The listing builds one solid part. Answer for the finished solid, in the listing's coordinates (mm). Face numbers are marked on the shaded views. Coordinates: 2 decimals unless noted, no trailing zeros. Order: outer loops, then holes, each group sorted by start corner. A loop starts at its lowest first (then second) coordinate and runs counter-clockwise, first axis right, second up. Notation, with made-up numbers: (38, 20.5) - (61, 20.5) arc R31 ccw to (61, 47.5) - close; hole circle Ø9 at (56, 36.5). An arc over 180 degrees is marked (long way). Use a Markdown table: item, result. Add a question column.
Item 1: The part is cut by section C-C, the plane y = -1.5. Give the vertices of the cut face in (x, z).
Item 2: The part is cut by section B-B, the plane x = 2.5. Give the vertices of the cut face in (y, z), then the cut area to 3 significant figures.
Item 3: Find the intervals of material crossed by line 1 along X through (y, z) = (-3.25, 9.5); line 2 along X through (y, z) = (-1, -2); line 3 along Y through (x, z) = (-2.75, 10.25), in increasing order.
Item 4: The part is cut by section D-D, the plane z = -1.5. Give the vertices of the cut face in (x, y), then the cut area to 3 significant figures.
Item 5: The mould has two halves that part along Z. Classify the marked faces 1, 2 and 3: released by +Z, released by -Z, zero draft, split by the parting line, or undercut.
Item 6: Flat-ended cylindrical pins translate along their axes: P1, Ø2, axis at y = -2, z = 0, coming from the +X side; P2, Ø1.6, axis at x = 5, y = -0.5, coming from the +Z side; P3, Ø4, axis at y = -2.5, z = 5, coming from the -X side. Find the tip coordinate at first contact, or state that the pin passes through.
Item 7: The part is cut by section A-A, the plane z = 11.75. Give the vertices of the cut face in (x, y).
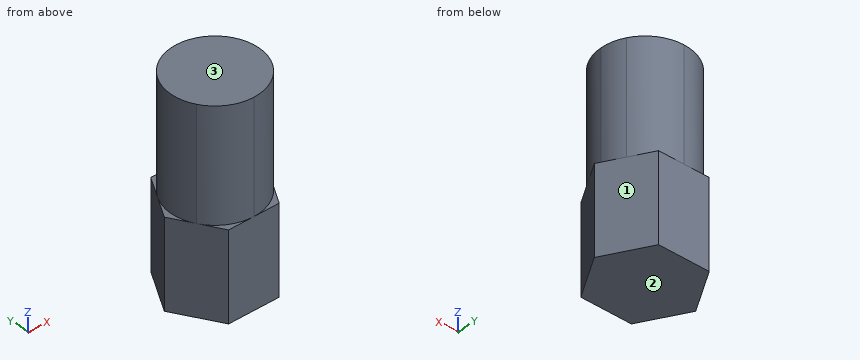
from build123d import *

# Parameters (mm, degrees)
F1_DEPTH = 5.0038
F3_DEPTH = 12.7


with BuildPart() as f1:
    # F0 (on Top) → F1 (new body, symmetric)
    with BuildSketch(Plane.XY):
        Polygon((2.888945, 5.0038), (-2.888945, 5.0038), (-5.777891, 0), (-2.888945, -5.0038), (2.888945, -5.0038), (5.777891, 0), align=None)
    extrude(amount=F1_DEPTH, both=True)

    # F2 (on face) → F3 (join)
    with BuildSketch(Plane.XY.offset(5.0038)):
        with BuildLine():
            ThreePointArc((4.333418, -2.5019), (4.8333, -1.295079), (5.0038, 0))
            ThreePointArc((5.0038, 0), (4.8333, 1.295079), (4.333418, 2.5019))
            ThreePointArc((4.333418, 2.5019), (2.5019, 4.333418), (0, 5.0038))
            ThreePointArc((0, 5.0038), (-2.5019, 4.333418), (-4.333418, 2.5019))
            ThreePointArc((-4.333418, 2.5019), (-5.0038, 0), (-4.333418, -2.5019))
            ThreePointArc((-4.333418, -2.5019), (-2.5019, -4.333418), (0, -5.0038))
            ThreePointArc((0, -5.0038), (2.5019, -4.333418), (4.333418, -2.5019))
        make_face()
    extrude(amount=F3_DEPTH)


solid = f1.part
Solution:
| question | item | result |
|---|---|---|
| 1 | outline | (-4.91, -5) - (4.91, -5) - (4.91, 5) - (4.77, 5) - (4.77, 17.7) - (-4.77, 17.7) - (-4.77, 5) - (-4.91, 5) - close |
| 2 | outline | (-5, -5) - (5, -5) - (5, 5) - (4.33, 5) - (4.33, 17.7) - (-4.33, 17.7) - (-4.33, 5) - (-5, 5) - close |
| 2 | area | 210 mm2 |
| 3 | line 1 | x = -3.8 to 3.8 |
| 3 | line 2 | x = -5.2 to 5.2 |
| 3 | line 3 | y = -4.18 to 4.18 |
| 4 | outline | (-5.78, 0) - (-2.89, -5) - (2.89, -5) - (5.78, 0) - (2.89, 5) - (-2.89, 5) - close |
| 4 | area | 86.7 mm2 |
| 5 | face 1 | zero draft |
| 5 | face 2 | released by -Z |
| 5 | face 3 | released by +Z |
| 6 | P1 | stops at x = 5.2 |
| 6 | P2 | stops at z = 17.7 |
| 6 | P3 | stops at x = -5.49 |
| 7 | outline | (4.33, -2.5) arc R5 ccw to (5, 0) arc R5 ccw to (4.33, 2.5) arc R5 ccw (long way) to start |
